Read the model definition and answer for the solid it produces. Units are mm, in the model's axes. A direction names the side the tool comes from. Give positions to 0.01 mm unless a question says otherwise; leave off trailing zeros. Order: outer loops, then holes, each group sorted by start corner. A loop starts at its lowest first (then second) coordinate and runs counter-clockwise, first axis right, second up.
Autodesk Inventor part; units mm, degrees
ref_plane "Work Plane1" through (0, 0, -4.25) normal (0, 0, 1) x (1, 0, 0)
ref_plane "Work Plane2" through (0, 0, -10.25) normal (0, 0, 1) x (1, 0, 0)
ref_plane "Work Plane5" through (0, 0, -5.125) normal (0, 0, -1) x (-1, 0, 0)
sketch "Sketch1" plane through (0, 0, 0) normal (0, 0, 1) x (1, 0, 0)
  circle A0 centre (0, 0) radius 29.9
  circle A1 centre (0, 0) radius 13.6
  dimension "d0" = 59.8
  dimension "d1" = 27.2
extrude "Extrusion1" add sketch "Sketch1" against normal blind 15
ref_plane "Work Plane1" through (0, 0, -4.25) normal (0, 0, 1) x (1, 0, 0)
ref_plane "Work Plane2" through (0, 0, -10.25) normal (0, 0, 1) x (1, 0, 0)
sketch "Sketch2" plane through (0, 0, 0) normal (0, 0, 1) x (1, 0, 0)
  circle A0 centre (0, 0) radius 29.9
  circle A1 centre (0, 0) radius 13.6
  circle A2 centre (0, 0) radius 12.6
  circle A3 centre (0, 0) radius 31.9
  dimension "d4" = 1
  dimension "d8" = 2
extrude "Extrusion2" add sketch "Sketch2" against normal up to surface (10.75 mm away) from surface at -4.25 contours A1
extrude "Extrusion3" add sketch "Sketch2" against normal up to surface (4.75 mm away) from surface at -10.25 contours A3
sketch "Sketch8" plane through (0, 0, 0) normal (0, 0, 1) x (1, 0, 0)
  circle A0 centre (0, 0) radius 29.9
  circle A1 centre (0, 0) radius 13.6
  circle A2 centre (0, 0) radius 31.9
  circle A3 centre (0, 0) radius 12.6
extrude "Extrusion8" add sketch "Sketch8" along normal blind 2 contours A0 | A1 | A2
sketch "Sketch9" plane through (0, 0, 2) normal (0, 0, 1) x (1, 0, 0)
  circle A0 centre (0, 0) radius 29.9
  circle A1 centre (0, 0) radius 29.9
  circle A2 centre (0, 0) radius 13.6
  circle A3 centre (0, 0) radius 13.6
  line L0 (0, 29.9) -> (0, 13.6) construction
  point P0 (0, 21.75)
hole "Hole3" at (0, 21.75, 2) direction (0, 0, -1) diameter 5.3 end through all
pattern_circular "Circular Pattern2" count 6 over 360 about axis through (0, 0, 0) along (0, 0, 1) of "Hole3"
chamfer "Chamfer1" distance 1 angle 45 2 edges at (-31.9, 0, 2) (-12.6, 0, 2)
ref_plane "Work Plane5" through (0, 0, -5.125) normal (0, 0, -1) x (-1, 0, 0)
properties part number "Spool Holder BAse" material "ABS Plastic"
1) Consider L1, parallel to Y at x = 17, z = -7.5; L2, parallel to Y at x = 2, z = -0.75; L3, parallel to X at y = 10, z = -4. Determine where each line is inside the solid, lowest interval first.
Final values:
L1: y = -24.6 to -12.79, -8.96 to 8.96, 12.79 to 24.6
L2: y = -29.83 to -23.49, -20.01 to -13.45, 13.45 to 20.01, 23.49 to 29.83
L3: x = -28.18 to -21.34, -16.33 to -9.22, 9.22 to 16.33, 21.34 to 28.18
2) Given pin 1 (2 mm diameter, centred on y = 12.5, z = -3, fed in from +X); pin 2 (8 mm diameter, centred on x = 0.5, y = -7.5, fed in from +Z); pin 3 (8 mm diameter, centred on x = -8.5, z = -5, fed in from +Y); pin 4 (10 mm diameter, centred on x = -4.5, z = -6.5, fed in from -Y), each flat-ended and moving along its own axis, determine where each tip first touches the part or whether it passes through.
Final values:
pin 1: stops at x = 27.6
pin 2: passes through
pin 3: stops at y = 29.56
pin 4: stops at y = -31.88
3) The part is cut by section D-D on z = -11.5. Determine the outline of the cut face in (x, y) (3 decimals).
Final values:
outline: circle Ø63.8 at (0, 0); hole circle Ø5.3 at (-18.836, -10.875); hole circle Ø5.3 at (-18.836, 10.875); hole circle Ø25.2 at (0, 0); hole circle Ø5.3 at (0, -21.75); hole circle Ø5.3 at (0, 21.75); hole circle Ø5.3 at (18.836, -10.875); hole circle Ø5.3 at (18.836, 10.875)
4) The part is cut by section A-A on y = 0. Determine the outline of the cut face in (x, z).
Final values:
outline: (-31.9, -15) - (-12.6, -15) - (-12.6, -4.25) - (-13.6, -4.25) - (-13.6, 0) - (-12.6, 0) - (-12.6, 1) - (-13.6, 2) - (-30.9, 2) - (-31.9, 1) - (-31.9, 0) - (-29.9, 0) - (-29.9, -10.25) - (-31.9, -10.25) - close; (12.6, -15) - (31.9, -15) - (31.9, -10.25) - (29.9, -10.25) - (29.9, 0) - (31.9, 0) - (31.9, 1) - (30.9, 2) - (13.6, 2) - (12.6, 1) - (12.6, 0) - (13.6, 0) - (13.6, -4.25) - (12.6, -4.25) - close
5) For a pull along Z with two mould halves and no side action, classify faces 1 (the face through (9, 29, 0)), 2 (the face through (6, -13, 2)), 3 (the face through (-2.948, -13.277, -2.095)), 4 (the face through (16.485, 12.098, -6.619)) as released by +Z, released by -Z, zero draft, split by the parting line, or undercut.
Final values:
face 1: undercut
face 2: released by +Z
face 3: undercut
face 4: zero draft
6) The part is cut by section B-B on z = -3.5. Determine the outline of the cut face in (x, y) (3 decimals), and give its area (3 significant figures).
Final values:
outline: circle Ø59.8 at (0, 0); hole circle Ø5.3 at (-18.836, -10.875); hole circle Ø5.3 at (-18.836, 10.875); hole circle Ø27.2 at (0, 0); hole circle Ø5.3 at (0, -21.75); hole circle Ø5.3 at (0, 21.75); hole circle Ø5.3 at (18.836, -10.875); hole circle Ø5.3 at (18.836, 10.875)
area: 2,100 mm2
7) The part is cut by section C-C on x = 0. Count the separate pieces of the cut face and the enclosed holes in it, and give its area (4 significant figures).
Final values:
separate pieces: 4
enclosed holes: 0
area: 424.5 mm2
8) A tool of negligible diameter and unlimited length cuts with its end or side. For faces 5 (the face through (9, 29, -10.25)), 6 (the face through (14, 0, -15)), from which of +Z, -Z, +X, -X, +Y, -Y can it reach the whole face along a straight path? Write none if from no direction.
Final values:
face 5: none
face 6: -Z, +X, -X, +Y, -Y
